```python
from build123d import *


with BuildPart() as part:
    # Esquisse1 → Base-Révolution (revolve)
    with BuildSketch(Plane.XY, mode=Mode.PRIVATE) as base_r_volution_sk:
        Polygon((0, 0), (0, 4.5), (2, 6.5), (8, 6.5), (8, 9), (12.5, 9), (12.5, 7.5), (20.5, 7.5), (20.5, 6.5), (36.5, 6.5), (36.5, 6), (46, 6), (46, 5), (47, 5), (47, 6), (49, 6), (50, 5), (50, 0), align=None)
    revolve(base_r_volution_sk.sketch.rotate(Axis((0, 0, 0), (1, 0, 0)), 90), axis=Axis((0, 0, 0), (1, 0, 0)))


solid = part.part
```
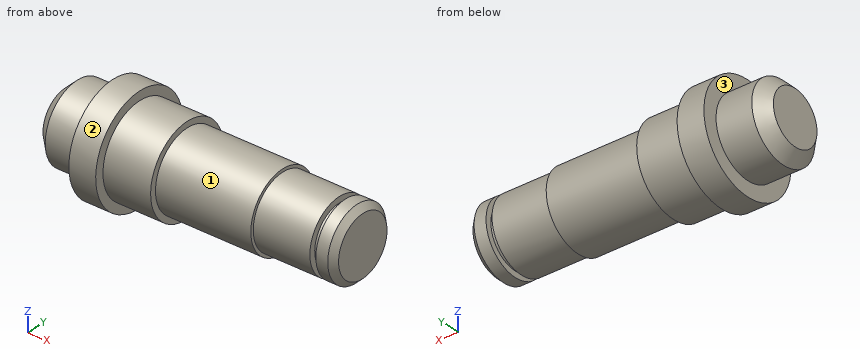
CAD build for the part. Positions are in the model's coordinates, mm. Face numbers are marked on the shaded views. A direction names the side the tool comes from. Round coordinates to 2 decimals unless told otherwise and drop trailing zeros. Loops run counter-clockwise (first coordinate to the right, second up) from the corner with the lowest first, then second, coordinate; pieces in that order, holes last. Notation, with made-up numbers: M -35,-6 L 14,-6 A22 ccw 14,2 Z; hole C 76,-14 d5. An arc over 180 degrees is marked long. Return JSON: item names as keys, results as strings. Group by question number.
(1) Saw through at D-D, the plane x = 30.5. List the corners of the cut face in (y, z), and give its area (3 significant figures).
(2) Wall check: probe 1 along X at (y, z) = (0.25, -7.25); probe 2 along Y at (x, z) = (15.5, 0.25); probe 3 along X at (y, z) = (5, 6.75). Give the ranges that are in metal, low to high. Write a range as [from, to].
(3) Tool access for the marked faces 1, 2 and 3: list every direction of +Z, -Z, +X, -X, +Y, -Y with a clear straight run to the whole face (end or side of a thin tool).
(4) Drop flat-ended pins along their axis: P1, Ø1.5, axis at x = 25, z = 0, coming from the +Y side; P2, Ø5, axis at x = 28, y = -3, coming from the +Z side; P3, Ø6, axis at x = 8, y = -5, coming from the -Z side. Give the stop position or say it passes through.
(5) Saw through at C-C, the plane x = 45. List the corners of the cut face in (y, z).
Answer list:
{
 "1": {"outline": "C 0,0 d13", "area": "133 mm2"},
 "2": {"probe 1": "[8, 20.5]", "probe 2": "[-7.5, 7.5]", "probe 3": "[8, 12.5]"},
 "3": {"face 1": "+X", "face 2": "+X, -X", "face 3": "-X"},
 "4": {"P1": "y = 6.5", "P2": "z = 6.48", "P3": "z = -8.77"},
 "5": {"outline": "C 0,0 d12"}
}
